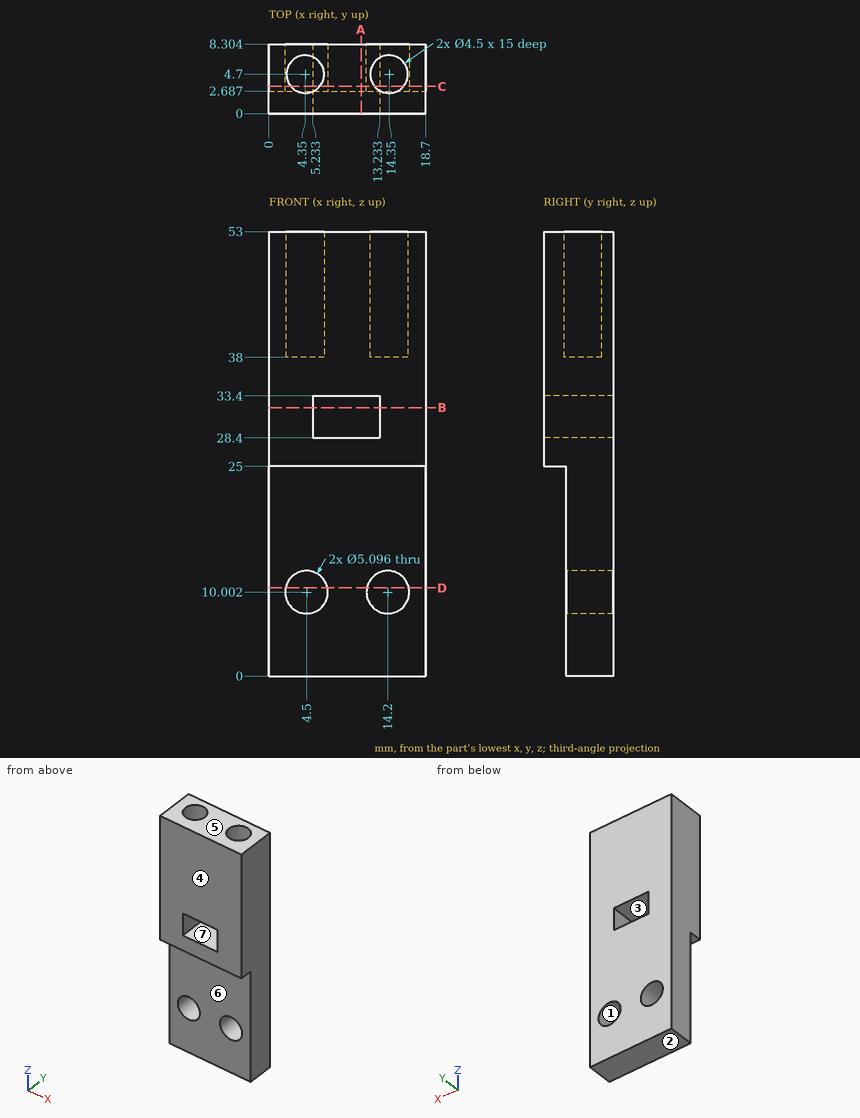
Answer from the drawing. Dimensions are ordinates in mm from the lowest x, y and z of the part. A direction names the side the tool comes from. Round coordinates to 2 decimals unless told otherwise and drop trailing zeros. Write each loop counter-clockwise with the first axis right and the second up, starting at its lowest first coordinate (ties: lowest second). Pieces come first, ordered by that corner, then holes. Notation, with made-up numbers: M -20,63 L -9,63 A11 cw -9,72 Z; hole C 75,57 d3. An arc over 180 degrees is marked long. Write each question's results on one line, items separated by ' | '. Start each with the question number.
Item 1: Given pin 1 Ø9.5 at (x, z) = (7.5, 16) entering from -Y; pin 2 Ø1.3 at (x, y) = (9.5, 1) entering from -Z; pin 3 Ø8 at (x, z) = (4.5, 10) entering from +Y; pin 4 Ø3.5 at (x, y) = (14.35, 4.7) entering from +Z, each flat-ended and moving along its own axis, determine where each tip first touches the part or whether it passes through.
Item 2: Which of the six approach directions +Z, -Z, +X, -X, +Y, -Y give full straight-line access (tool end or side, diameter ignored) to the marked faces 5, 6 and 7?
Item 3: Straight lines are drawn through the part: probe 1 along X at (y, z) = (6.5, 10); probe 2 along Z at (x, y) = (14.2, 5.5); probe 3 along Z at (x, y) = (9.5, 1.5). For each, find the intervals that lie inside material, in ascending order.
Item 4: Find section A-A on x = 11. Write down the section's boundary in (y, z) (1 decimal).
Item 5: Find section B-B on z = 32. Write down the section's boundary in (x, y) (1 decimal).
Item 6: Find section D-D on z = 10.5. Write down the section's boundary in (x, y) (1 decimal), and give its area (3 significant figures).
Item 7: The mould has two halves that part along Z. Classify the marked faces 1, 2, 3 and 4: +Z half, -Z half, draft (parallel to the pull), parting line (faces both ways), or undercut.
Item 8: Find section C-C on y = 3.25. Write down the section's boundary in (x, z), and give its area (3 significant figures).
Answer block:
1) pin 1: stops at y = 2.69 | pin 2: stops at z = 25 | pin 3: stops at y = 8.3 | pin 4: stops at z = 38
2) face 5: +Z, +X, -X, +Y, -Y | face 6: -Z, +X, -X, -Y | face 7: +Y, -Y
3) probe 1: x = 0 to 1.95, 7.05 to 11.65, 16.75 to 18.7 | probe 2: z = 0 to 7.45, 12.55 to 38 | probe 3: z = 25 to 28.4, 33.4 to 53
4) outline: M 0,25 L 2.7,25 L 2.7,0 L 8.3,0 L 8.3,28.4 L 0,28.4 Z; M 0,33.4 L 8.3,33.4 L 8.3,53 L 0,53 Z
5) outline: M 0,0 L 5.2,0 L 5.2,8.3 L 0,8.3 Z; M 13.2,0 L 18.7,0 L 18.7,8.3 L 13.2,8.3 Z
6) outline: M 0,2.7 L 2,2.7 L 2,8.3 L 0,8.3 Z; M 7,2.7 L 11.7,2.7 L 11.7,8.3 L 7,8.3 Z; M 16.7,2.7 L 18.7,2.7 L 18.7,8.3 L 16.7,8.3 Z | area: 48.9 mm²
7) face 1: undercut | face 2: -Z half | face 3: undercut | face 4: draft
8) outline: M 0,0 L 18.7,0 L 18.7,53 L 16.07,53 L 16.07,38 L 12.63,38 L 12.63,53 L 6.07,53 L 6.07,38 L 2.63,38 L 2.63,53 L 0,53 Z; hole C 4.5,10 d5.1; hole M 5.23,28.4 L 13.23,28.4 L 13.23,33.4 L 5.23,33.4 Z; hole C 14.2,10 d5.1 | area: 807 mm²
